Part print with two shaded views. Sizes in mm from the minimum x, y, z corner. A direction names the side the tool comes from. Coordinates: 2 decimals unless noted, no trailing zeros. Write each loop counter-clockwise with the first axis right and the second up, starting at its lowest first coordinate (ties: lowest second). Pieces come first, ordered by that corner, then holes. Notation, with made-up numbers: (18, 86.5) - (55, 86.5) arc R27 cw to (55, 114.5) - close; hole circle Ø10 at (35.5, -13.75). An arc over 180 degrees is marked (long way). One line per question, with ' | ' between items. Start each with the question number.
1. Band-saw the part on B-B, the plane x = 31.5. Write the cut outline in (y, z), then the cut area to 3 significant figures.
2. Flat gauge pins, fed straight in: P1, Ø3, axis at y = 19, z = 7, coming from the -X side; P2, Ø3, axis at x = 28, z = 5, coming from the -Y side; P3, Ø6, axis at x = 91, z = 5, coming from the -Y side. Where does each tip first touch, or does it go through?
3. Which spindle directions (+Z, -Z, +X, -X, +Y, -Y) get a long thin tool onto all of the face, cutting with end or side? Do the marked faces 1 and 2. Say none if no direction does.
4. Band-saw the part on A-A, the plane z = 1.5. Write the cut outline in (x, y).
5. Band-saw the part on C-C, the plane y = 30.5. Write the cut outline in (x, z).
6. Probe line 1 (Y direction, x = 32, z = 4); line 2 (X direction, y = 23, z = 2). List the from-to ranges inside material, lowest first.
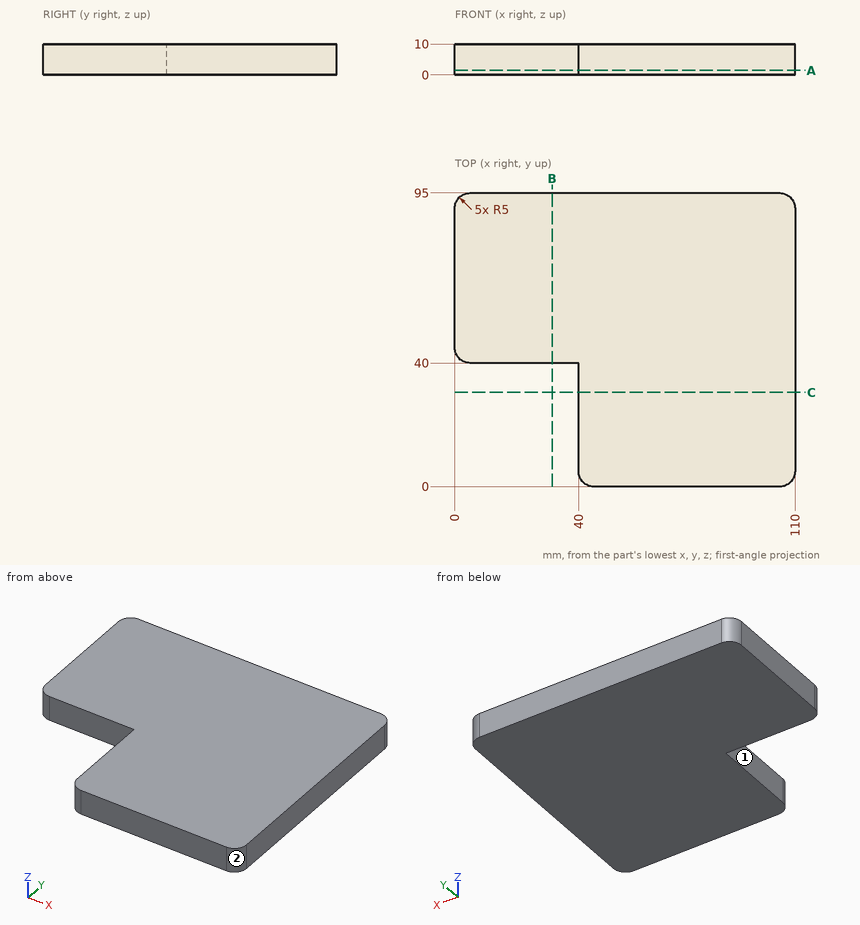
Filled in:
1) outline: (40, 0) - (95, 0) - (95, 10) - (40, 10) - close | area: 550 mm²
2) P1: stops at x = 40 | P2: stops at y = 40 | P3: stops at y = 0
3) face 1: +Z, -Z, -X, -Y | face 2: +Z, -Z, +X, -Y
4) outline: (0, 45) arc R5 ccw to (5, 40) - (40, 40) - (40, 5) arc R5 ccw to (45, 0) - (105, 0) arc R5 ccw to (110, 5) - (110, 90) arc R5 ccw to (105, 95) - (5, 95) arc R5 ccw to (0, 90) - close
5) outline: (40, 0) - (110, 0) - (110, 10) - (40, 10) - close
6) line 1: y = 40 to 95 | line 2: x = 40 to 110
